For this review, take the finished solid that the model builds, in its own axes (mm). A direction names the side the tool comes from. Give positions to 0.01 mm unless a question says otherwise; leave off trailing zeros. Order: outer loops, then holes, each group sorted by start corner. A loop starts at its lowest first (then second) coordinate and runs counter-clockwise, first axis right, second up. Notation, with made-up numbers: M 39,25.5 L 91,25.5 A22 cw 91,44.5 Z; hole C -1,-10 d3. An arc over 180 degrees is marked long. Answer as CSV lines item,"result". Start each with the question number.
1. Clearance check with a flat-ended pin moving along its axis: P1, Ø2.5, axis at x = 27.5, z = 4.5, coming from the +Y side. State where the tip first meets the part, or that it passes through.
2. We need section A-A, the plane y = 7.5. Give the boundary of the cut face in (x, z).
3. We need section B-B, the plane x = 20. Give the boundary of the cut face in (y, z).
4. We need section D-D, the plane x = 25.5. Give the boundary of the cut face in (y, z), and give its area (3 significant figures).
5. Mouldability with a two-part tool opening along Y and no side actions: class faces 1 (the flat face through (18.6, 32.5, 8)), 2 (the cylindrical face through (7.43, 20.6, 3.94)), 3 (the cylindrical face through (38.797, 34.859, 3.042)) as pulls with the +Y half, pulls with the -Y half, needs draft (parallel to the pull), parting line crosses it, or undercut.
6. For line 1 along X through (y, z) = (17, 5.75); line 2 along Z through (x, y) = (20, 37); line 3 along Y through (x, z) = (26, 2.5), list the stretches that pass through material, from the lowest coordinate up.
7. Machinability: for faces 4 (the flat face through (35, 20, 4)), 5 (the flat face through (23, 33, 4)), 6 (the flat face through (30, 36, 3)), 7 (the cylindrical face through (39.43, 18.2, 7.4)), 8 (the cylindrical face through (28.9, 35.43, 7.4)), which of the approach directions +Z, -Z, +X, -X, +Y, -Y give a long, thin tool a straight path to every point of the face, cutting with its end or side? Answer none if there is none.
from build123d import *

# Parameters (mm, degrees)
SKETCH_W        = 40
SKETCH_H        = 36
PAD_DEPTH       = 8
POCKET_DEPTH    = 8
FILLET_R        = 4
FILLET001_R     = 4
FILLET002_R     = 4
FILLET003_R     = 4
SKETCH002_W     = 8
SKETCH002_H     = 8
PAD001_DEPTH    = 6
FILLET004_R     = 2
FILLET005_R     = 2
FILLET006_R     = 2
FILLET007_R     = 2
FILLET008_R     = 2
SKETCH003_R     = 2
POCKET001_DEPTH = 10
SKETCH004_W     = 6
SKETCH004_H     = 6
POCKET002_DEPTH = 1.5


with BuildPart() as part:
    # Sketch → Pad (new body)
    with BuildSketch(Plane.XY):
        with Locations((20, 18)):
            Rectangle(SKETCH_W, SKETCH_H)
    extrude(amount=PAD_DEPTH)

    # Sketch001 → Pocket (cut)
    with BuildSketch(Plane.XY.offset(8)):
        Polygon((4, 4), (4, 20), (8, 20), (8, 32), (32, 32), (32, 20), (36, 20), (36, 4), align=None)
    extrude(amount=-POCKET_DEPTH, mode=Mode.SUBTRACT)

    # Fillet
    fillet_edges = [part.edges().sort_by_distance(p)[0] for p in [
        (40, 36, 4),
    ]]
    fillet(fillet_edges, radius=FILLET_R)

    # Fillet001
    fillet001_edges = [part.edges().sort_by_distance(p)[0] for p in [
        (0, 36, 4),
    ]]
    fillet(fillet001_edges, radius=FILLET001_R)

    # Fillet002
    fillet002_edges = [part.edges().sort_by_distance(p)[0] for p in [
        (40, 0, 4),
    ]]
    fillet(fillet002_edges, radius=FILLET002_R)

    # Fillet003
    fillet003_edges = [part.edges().sort_by_distance(p)[0] for p in [
        (0, 0, 4),
    ]]
    fillet(fillet003_edges, radius=FILLET003_R)

    # Sketch002 → Pad001 (new body)
    with BuildSketch(Plane(origin=(0, 36, 0), x_dir=(-1, 0, 0), z_dir=(0, 1, 0))):
        with Locations((-20, 4)):
            Rectangle(SKETCH002_W, SKETCH002_H)
    extrude(amount=PAD001_DEPTH)

    # Fillet004
    fillet004_edges = [part.edges().sort_by_distance(p)[0] for p in [
        (40, 18, 8),
    ]]
    fillet(fillet004_edges, radius=FILLET004_R)

    # Fillet005
    fillet005_edges = [part.edges().sort_by_distance(p)[0] for p in [
        (8, 20, 4),
    ]]
    fillet(fillet005_edges, radius=FILLET005_R)

    # Fillet006
    fillet006_edges = [part.edges().sort_by_distance(p)[0] for p in [
        (32, 20, 4),
    ]]
    fillet(fillet006_edges, radius=FILLET006_R)

    # Fillet007
    fillet007_edges = [part.edges().sort_by_distance(p)[0] for p in [
        (24, 39, 8),
    ]]
    fillet(fillet007_edges, radius=FILLET007_R)

    # Fillet008
    fillet008_edges = [part.edges().sort_by_distance(p)[0] for p in [
        (16, 39, 8),
    ]]
    fillet(fillet008_edges, radius=FILLET008_R)

    # Sketch003 → Pocket001 (cut)
    with BuildSketch(Plane(origin=(0, 42, 0), x_dir=(-1, 0, 0), z_dir=(0, 1, 0))):
        with Locations((-20, 4)):
            Circle(SKETCH003_R)
    extrude(amount=-POCKET001_DEPTH, mode=Mode.SUBTRACT)

    # Sketch004 → Pocket002 (cut)
    with BuildSketch(Plane.XZ.offset(-32)):
        with Locations((20, 4)):
            Rectangle(SKETCH004_W, SKETCH004_H)
    extrude(amount=-POCKET002_DEPTH, mode=Mode.SUBTRACT)


solid = part.part
Result set:
1,P1,"y = 36"
2,outline,"M 0,0 L 4,0 L 4,8 L 2,8 A2 ccw 0,6 Z; M 36,0 L 40,0 L 40,6 A2 ccw 38,8 L 36,8 Z"
3,outline,"M 0,0 L 4,0 L 4,8 L 2,8 A2 ccw 0,6 Z; M 32,0 L 42,0 L 42,2 L 33.5,2 L 33.5,1 L 32,1 Z; M 32,7 L 33.5,7 L 33.5,6 L 42,6 L 42,8 L 32,8 Z"
4,outline,"M 0,0 L 4,0 L 4,8 L 2,8 A2 ccw 0,6 Z; M 32,0 L 36,0 L 36,6 A2 ccw 34,8 L 32,8 Z"
4,area,"62.3 mm2"
5,face 1,"needs draft"
5,face 2,"undercut"
5,face 3,"pulls with the +Y half"
6,line 1,"0 to 4, 36 to 40"
6,line 2,"0 to 2, 6 to 8"
6,line 3,"0 to 4, 32 to 36"
7,face 4,"+Z, -Z"
7,face 5,"none"
7,face 6,"+Z, -Z, +X, +Y"
7,face 7,"+Z, +X, +Y, -Y"
7,face 8,"+Z, +X, +Y"
